Geometry check sheet. Reference: the model listing, model coordinates, mm. Give positions to 0.01 mm unless a question says otherwise; leave off trailing zeros. Order: outer loops, then holes, each group sorted by start corner. A loop starts at its lowest first (then second) coordinate and runs counter-clockwise, first axis right, second up. Notation, with made-up numbers: M -40,45.25 L -34,45.25 A10 ccw -34,54.25 Z; hole C 7.25,-12.75 d7. An arc over 180 degrees is marked long. Answer as CSV lines item,"result".
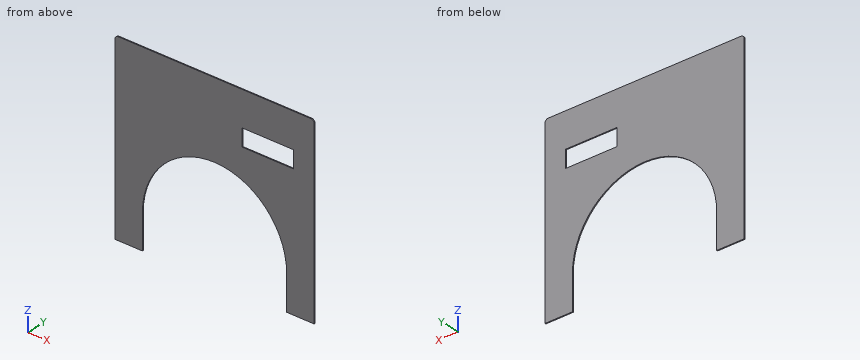
from build123d import *

# Parameters (mm, degrees)
F1_DEPTH = 3


with BuildPart() as f1:
    # F0 (on Front) → F1 (new body)
    with BuildSketch(Plane.XZ):
        with BuildLine():
            Line((280, 430), (-280, 430))
            ThreePointArc((-280, 430), (-287.071068, 427.071068), (-290, 420))
            Line((-290, 420), (-290, -100))
            Line((-290, -100), (-210, -100))
            Line((-210, -100), (-210, 0))
            ThreePointArc((-210, 0), (-148.454947, 148.529892), (0.105988, 209.999973))
            ThreePointArc((0.105988, 209.999973), (148.529892, 148.454947), (210, 0))
            Line((210, 0), (210, -100))
            Line((210, -100), (290, -100))
            Line((290, -100), (290, 420))
            ThreePointArc((290, 420), (287.071068, 427.071068), (280, 430))
        make_face()
        Polygon((230, 280), (80, 280), (80, 329.965293), (230, 330), align=None, mode=Mode.SUBTRACT)
    extrude(amount=F1_DEPTH)


solid = f1.part
(1) Section check D-D on x = 30. Enter the section's corners in (y, z).
The answers:
outline,"M -3,207.85 L 0,207.85 L 0,430 L -3,430 Z"
(2) Material ranges on line 1 (X direction, y = -2.4, z = -7); line 2 (X direction, y = -2.6, z = 191.5); line 3 (Z direction, x = 116, y = -0.95), recorded low to high.
The answers:
line 1,"x = -290 to -210, 210 to 290"
line 2,"x = -290 to -86.18, 86.18 to 290"
line 3,"z = 175.05 to 280, 329.97 to 430"
(3) Section check A-A on y = -2.3. Enter the section's corners in (x, z).
The answers:
outline,"M -290,-100 L -210,-100 L -210,0 A210 cw 0.11,210 A210 cw 210,0 L 210,-100 L 290,-100 L 290,420 A10 ccw 280,430 L -280,430 A10 ccw -290,420 Z; hole M 80,280 L 230,280 L 230,330 L 80,329.97 Z"
(4) Section check B-B on x = 98. Enter the section's corners in (y, z).
The answers:
outline,"M -3,185.73 L 0,185.73 L 0,280 L -3,280 Z; M -3,329.97 L 0,329.97 L 0,430 L -3,430 Z"
(5) Section check C-C on z = 52. Enter the section's corners in (x, y).
The answers:
outline,"M -290,-3 L -203.46,-3 L -203.46,0 L -290,0 Z; M 203.46,-3 L 290,-3 L 290,0 L 203.46,0 Z"
